CAD build for the part. Positions are in the model's coordinates, mm. A direction names the side the tool comes from. Round coordinates to 2 decimals unless told otherwise and drop trailing zeros. Loops run counter-clockwise (first coordinate to the right, second up) from the corner with the lowest first, then second, coordinate; pieces in that order, holes last.
```python
from build123d import *
from build123d.topology import SkipClean

# Parameters (mm, degrees)
BOSS_EXTRUDE1_DEPTH             = 10
BOSS_EXTRUDE2_DEPTH             = 1
BOSS_EXTRUDE3_DEPTH             = 7
CUT_EXTRUDE1_REACH              = 22.186
CUT_EXTRUDE2_REACH              = 22.166
BOSS_EXTRUDE4_REACH             = 24.566
BOSS_EXTRUDE4_END_RADIUS        = 3.5
SKETCH6_W                       = 5
SKETCH6_H                       = 3.45
SKETCH6_W_2                     = 3.2
SKETCH6_H_2                     = 1.65
BOSS_EXTRUDE4_DIRECTION_2_DEPTH = 19
CUT_EXTRUDE3_REACH              = 32.254
CUT_EXTRUDE4_REACH              = 32.254
CUT_EXTRUDE5_REACH              = 30.604


with BuildPart() as part:
    # Sketch1 → Boss-Extrude1 (new body)
    with BuildSketch(Plane(origin=(0, 0, 0), x_dir=(1, 0, 0), z_dir=(0, 1, 0))):
        with BuildLine():
            Line((-7.414489618, 1.20663528), (-4.430578599, 0.893013594))
            ThreePointArc((-4.430578599, 0.893013594), (-4.262003609, 0.936193276), (-4.162443929, 1.078916372))
            ThreePointArc((-4.162443929, 1.078916372), (-3.040559159, 3.040559159), (-1.078916372, 4.162443929))
            ThreePointArc((-1.078916372, 4.162443929), (-0.936193276, 4.262003609), (-0.893013594, 4.430578599))
            Line((-0.893013594, 4.430578599), (-1.20663528, 7.414489618))
            Line((-1.20663528, 7.414489618), (-0.361291669, 7.503338812))
            Line((-0.361291669, 7.503338812), (-0.047669983, 4.519427793))
            ThreePointArc((-0.047669983, 4.519427793), (0.02961483, 4.363514132), (0.189918705, 4.29580387))
            ThreePointArc((0.189918705, 4.29580387), (3.856330167, 1.902292734), (3.524282323, -2.463622152))
            Line((3.524282323, -2.463622152), (2.947715037, -1.887054865))
            ThreePointArc((2.947715037, -1.887054865), (-2.474873734, 2.474873734), (1.887054865, -2.947715037))
            Line((1.887054865, -2.947715037), (2.463622152, -3.524282323))
            ThreePointArc((2.463622152, -3.524282323), (-1.902292734, -3.856330167), (-4.29580387, -0.189918705))
            ThreePointArc((-4.29580387, -0.189918705), (-4.363514132, -0.02961483), (-4.519427793, 0.047669983))
            Line((-4.519427793, 0.047669983), (-7.503338812, 0.361291669))
            Line((-7.503338812, 0.361291669), (-7.414489618, 1.20663528))
        make_face()
    extrude(amount=-BOSS_EXTRUDE1_DEPTH)

    # Sketch2 → Boss-Extrude2 (add)
    with BuildSketch(Plane(origin=(0, -8.25, 0), x_dir=(-1, 0, 0), z_dir=(0, -1, 0))):
        with BuildLine():
            Line((-1.887054865, -2.947715037), (-1.15601211, -2.216672281))
            ThreePointArc((-1.15601211, -2.216672281), (1.767766953, 1.767766953), (-2.216672281, -1.15601211))
            Line((-2.216672281, -1.15601211), (-2.947715037, -1.887054865))
            ThreePointArc((-2.947715037, -1.887054865), (2.474873734, 2.474873734), (-1.887054865, -2.947715037))
        make_face()
    extrude(amount=BOSS_EXTRUDE2_DEPTH)

    # Sketch3 → Boss-Extrude3 (add)
    with SkipClean():  # the faces are left unmerged after this step: merging them gives an invalid solid
        with BuildSketch(Plane.XZ.offset(10)):
            with BuildLine():
                Line((-7.503338812, -0.361291669), (-3.499493713, 0.059529408))
                ThreePointArc((-3.499493713, 0.059529408), (-3.480826634, -0.365849621), (-3.41064452, -0.785814203))
                Line((-3.41064452, -0.785814203), (-7.414489618, -1.20663528))
                Line((-7.414489618, -1.20663528), (-7.503338812, -0.361291669))
            make_face()
            with BuildLine():
                Line((-1.20663528, -7.414489618), (-0.785814203, -3.41064452))
                ThreePointArc((-0.785814203, -3.41064452), (-0.365849621, -3.480826634), (0.059529408, -3.499493713))
                Line((0.059529408, -3.499493713), (-0.361291669, -7.503338812))
                Line((-0.361291669, -7.503338812), (-1.20663528, -7.414489618))
            make_face()
        extrude(amount=BOSS_EXTRUDE3_DEPTH)

    # Sketch4 → Cut-Extrude1 (cut, up to next)
    with BuildSketch(Plane(origin=(-0.044424597, 0, 0.422671806), x_dir=(0.9945218953682731, 0, 0.10452846326765693), z_dir=(-0.10452846326765693, 0, 0.9945218953682731)), mode=Mode.PRIVATE) as cut_extrude1_sk1:
        with BuildLine():
            Line((-4.499652764, 0), (-6.450238257, 0))
            ThreePointArc((-6.450238257, 0), (-7.174298022, -0.310262762), (-7.449060221, -1.048525086))
            Line((-7.449060221, -1.048525086), (-6.720325459, -16.048525086))
            ThreePointArc((-6.720325459, -16.048525086), (-6.411240733, -16.724059765), (-5.721503495, -17))
            Line((-5.721503495, -17), (-3.474100603, -17))
            Line((-3.474100603, -17), (-3.474100603, -18.237576525))
            Line((-3.474100603, -18.237576525), (-8.636241127, -18.237576525))
            Line((-8.636241127, -18.237576525), (-8.636241127, 0.642542217))
            Line((-8.636241127, 0.642542217), (-4.499652764, 0.642542217))
            Line((-4.499652764, 0.642542217), (-4.499652764, 0))
        make_face()
    cut_extrude1_tool1 = extrude(cut_extrude1_sk1.sketch, amount=-CUT_EXTRUDE1_REACH, mode=Mode.PRIVATE) & part.part
    add(cut_extrude1_tool1.solids().sort_by_distance((-7.422183, -10.016233, -0.352762))[0], mode=Mode.SUBTRACT)

    # Sketch5 → Cut-Extrude2 (cut, up to next)
    with BuildSketch(Plane(origin=(0.422671806, 0, -0.044424597), x_dir=(-0.10452846326764693, 0, -0.9945218953682741), z_dir=(0.9945218953682741, 0, -0.10452846326764693)), mode=Mode.PRIVATE) as cut_extrude2_sk1:
        with BuildLine():
            Line((4.499652764, 0), (6.39817036, 0))
            ThreePointArc((6.39817036, 0), (7.158143292, -0.325651711), (7.446533622, -1.100531645))
            Line((7.446533622, -1.100531645), (6.7226182, -16.001332189))
            ThreePointArc((6.7226182, -16.001332189), (6.398202955, -16.710373204), (5.674254938, -17))
            Line((5.674254938, -17), (3.474100603, -17))
            Line((3.474100603, -17), (3.474100603, -17.961134023))
            Line((3.474100603, -17.961134023), (9.689471059, -17.961134023))
            Line((9.689471059, -17.961134023), (9.520710585, 0.644708136))
            Line((9.520710585, 0.644708136), (4.499652764, 0.644708136))
            Line((4.499652764, 0.644708136), (4.499652764, 0))
        make_face()
    cut_extrude2_tool1 = extrude(cut_extrude2_sk1.sketch, amount=-CUT_EXTRUDE2_REACH, mode=Mode.PRIVATE) & part.part
    add(cut_extrude2_tool1.solids().sort_by_distance((-0.417746, -9.418745, -8.040463))[0], mode=Mode.SUBTRACT)

    # Boss-Extrude4: up to this cylinder (the profile starts outside it)
    with SkipClean():  # the faces are left unmerged after this step: merging them gives an invalid solid
        boss_extrude4_end = Plane(origin=(0, -1.260747, 0), z_dir=(0, 1, 0)) * Cylinder(BOSS_EXTRUDE4_END_RADIUS, 57.132, mode=Mode.PRIVATE)
        # Sketch6 → Boss-Extrude4 (add, up to the surface)
        with BuildSketch(Plane(origin=(3.040559159, 0, 3.040559159), x_dir=(0.7071067811865511, 0, -0.707106781186544), z_dir=(0.707106781186544, 0, 0.7071067811865511)), mode=Mode.PRIVATE) as boss_extrude4_sk1:
            with Locations((0, -2.925)):
                Rectangle(SKETCH6_W, SKETCH6_H)
            with Locations((0, -2.925)):
                Rectangle(SKETCH6_W_2, SKETCH6_H_2, mode=Mode.SUBTRACT)
        boss_extrude4_tool1 = extrude(boss_extrude4_sk1.sketch, amount=-BOSS_EXTRUDE4_REACH, mode=Mode.PRIVATE) - boss_extrude4_end
        add(boss_extrude4_tool1.solids().sort_by_distance((3.040559, -1.260747, 3.040559))[0])

    # Sketch6 → Boss-Extrude4 direction 2 (add)
    with SkipClean():  # the faces are left unmerged after this step: merging them gives an invalid solid
        with BuildSketch(Plane(origin=(3.040559159, 0, 3.040559159), x_dir=(0.7071067811865511, 0, -0.707106781186544), z_dir=(0.707106781186544, 0, 0.7071067811865511))):
            with Locations((0, -2.925)):
                Rectangle(SKETCH6_W, SKETCH6_H)
            with Locations((0, -2.925)):
                Rectangle(SKETCH6_W_2, SKETCH6_H_2, mode=Mode.SUBTRACT)
        extrude(amount=BOSS_EXTRUDE4_DIRECTION_2_DEPTH)

    # Sketch7 → Cut-Extrude3 (cut, up to next)
    with BuildSketch(Plane(origin=(0, -1.2, 0), x_dir=(1, 0, 0), z_dir=(0, 1, 0)), mode=Mode.PRIVATE) as cut_extrude3_sk1:
        with BuildLine():
            Line((15.344217152, -17.606958852), (13.965358928, -16.228100628))
            ThreePointArc((13.965358928, -16.228100628), (13.511374439, -15.132085117), (13.965358928, -14.036069607))
            Line((13.965358928, -14.036069607), (14.036069607, -13.965358928))
            ThreePointArc((14.036069607, -13.965358928), (15.132085117, -13.511374439), (16.228100628, -13.965358928))
            Line((16.228100628, -13.965358928), (17.606958852, -15.344217152))
            Line((17.606958852, -15.344217152), (15.344217152, -17.606958852))
        make_face()
    cut_extrude3_tool1 = extrude(cut_extrude3_sk1.sketch, amount=-CUT_EXTRUDE3_REACH, mode=Mode.PRIVATE) & part.part
    # Sketch7 → Cut-Extrude3 (cut, up to next)
    with BuildSketch(Plane(origin=(0, -1.2, 0), x_dir=(1, 0, 0), z_dir=(0, 1, 0)), mode=Mode.PRIVATE) as cut_extrude3_sk2:
        Polygon((8.379215357, -10.641957057), (10.641957057, -8.379215357), (13.116830791, -10.854089091), (10.854089091, -13.116830791), align=None)
    cut_extrude3_tool2 = extrude(cut_extrude3_sk2.sketch, amount=-CUT_EXTRUDE3_REACH, mode=Mode.PRIVATE) & part.part
    # Sketch7 → Cut-Extrude3 (cut, up to next)
    with BuildSketch(Plane(origin=(0, -1.2, 0), x_dir=(1, 0, 0), z_dir=(0, 1, 0)), mode=Mode.PRIVATE) as cut_extrude3_sk3:
        Polygon((3.924442636, -6.187184335), (6.187184335, -3.924442636), (8.591347391, -6.328605692), (6.328605692, -8.591347391), align=None)
    cut_extrude3_tool3 = extrude(cut_extrude3_sk3.sketch, amount=-CUT_EXTRUDE3_REACH, mode=Mode.PRIVATE) & part.part
    add(cut_extrude3_tool1.solids().sort_by_distance((15.338807, -1.2, 15.338807))[0], mode=Mode.SUBTRACT)
    add(cut_extrude3_tool2.solids().sort_by_distance((10.748023, -1.2, 10.748023))[0], mode=Mode.SUBTRACT)
    add(cut_extrude3_tool3.solids().sort_by_distance((6.257895, -1.2, 6.257895))[0], mode=Mode.SUBTRACT)

    # Cut-Extrude4: up to this face of the body (flat: up to its plane)
    cut_extrude4_end = Plane(part.part.faces().sort_by_distance((9.75807358, -4.65, 9.75807358))[0])
    # Sketch8 → Cut-Extrude4 (cut, up to the picked face)
    with BuildSketch(Plane(origin=(0, -1.2, 0), x_dir=(1, 0, 0), z_dir=(0, 1, 0)), mode=Mode.PRIVATE) as cut_extrude4_sk1:
        with BuildLine():
            Line((1.887054865, -2.947715037), (2.463622152, -3.524282323))
            ThreePointArc((2.463622152, -3.524282323), (2.122539393, -3.739629196), (1.762778319, -3.922067388))
            Line((1.762778319, -3.922067388), (1.894971957, -4.082617205))
            ThreePointArc((1.894971957, -4.082617205), (2.256834016, -4.264215104), (2.634518611, -4.118351149))
            Line((2.634518611, -4.118351149), (4.118351149, -2.634518611))
            ThreePointArc((4.118351149, -2.634518611), (4.264215104, -2.256834016), (4.082617205, -1.894971957))
            Line((4.082617205, -1.894971957), (3.922067388, -1.762778319))
            ThreePointArc((3.922067388, -1.762778319), (3.739629196, -2.122539393), (3.524282323, -2.463622152))
            Line((3.524282323, -2.463622152), (2.947715037, -1.887054865))
            ThreePointArc((2.947715037, -1.887054865), (2.474873734, -2.474873734), (1.887054865, -2.947715037))
        make_face()
    cut_extrude4_tool1 = split(extrude(cut_extrude4_sk1.sketch, amount=-CUT_EXTRUDE4_REACH, mode=Mode.PRIVATE), bisect_by=cut_extrude4_end, keep=Keep.BOTH, mode=Mode.PRIVATE)
    add(cut_extrude4_tool1.solids().sort_by(Axis((2.984609, -1.2, 2.984609), (0, -1, 0)))[0], mode=Mode.SUBTRACT)

    # Sketch9 → Cut-Extrude5 (cut, up to next)
    with BuildSketch(Plane.XZ.offset(4.65), mode=Mode.PRIVATE) as cut_extrude5_sk1:
        Polygon((9.75807358, 12.02081528), (12.02081528, 9.75807358), (17.606958852, 15.344217152), (15.344217152, 17.606958852), align=None)
    cut_extrude5_tool1 = extrude(cut_extrude5_sk1.sketch, amount=-CUT_EXTRUDE5_REACH, mode=Mode.PRIVATE) & part.part
    # Sketch9 → Cut-Extrude5 (cut, up to next)
    with BuildSketch(Plane.XZ.offset(4.65), mode=Mode.PRIVATE) as cut_extrude5_sk2:
        Polygon((8.485281374, 10.748023074), (10.748023074, 8.485281374), (8.27314934, 6.01040764), (6.01040764, 8.27314934), align=None)
    cut_extrude5_tool2 = extrude(cut_extrude5_sk2.sketch, amount=-CUT_EXTRUDE5_REACH, mode=Mode.PRIVATE) & part.part
    # Sketch9 → Cut-Extrude5 (cut, up to next)
    with BuildSketch(Plane.XZ.offset(4.65), mode=Mode.PRIVATE) as cut_extrude5_sk3:
        Polygon((2.952170811, 5.214912511), (5.214912511, 2.952170811), (7.000357134, 4.737615434), (4.737615434, 7.000357134), align=None)
    cut_extrude5_tool3 = extrude(cut_extrude5_sk3.sketch, amount=-CUT_EXTRUDE5_REACH, mode=Mode.PRIVATE) & part.part
    add(cut_extrude5_tool1.solids().sort_by_distance((13.682516, -4.65, 13.682516))[0], mode=Mode.SUBTRACT)
    add(cut_extrude5_tool2.solids().sort_by_distance((8.379215, -4.65, 8.379215))[0], mode=Mode.SUBTRACT)
    add(cut_extrude5_tool3.solids().sort_by_distance((4.976264, -4.65, 4.976264))[0], mode=Mode.SUBTRACT)


solid = part.part
```
Item 1: Cut at D-D, the plane y = -7.25. Give the cut face in (x, z).
Answers follow:
outline: (-7.15, -0.32) - (-7.06, -1.17) - (-4.43, -0.89) arc R0.25 cw to (-4.16, -1.08) arc R4.3 ccw to (-1.08, -4.16) arc R0.25 cw to (-0.89, -4.43) - (-1.17, -7.06) - (-0.32, -7.15) - (-0.05, -4.52) arc R0.25 cw to (0.19, -4.3) arc R4.3 ccw to (3.52, 2.46) - (2.95, 1.89) arc R3.5 cw (long way) to (1.89, 2.95) - (2.46, 3.52) arc R4.3 ccw to (-4.3, 0.19) arc R0.25 cw to (-4.52, -0.05) - close
Item 2: Probe line 1 (Y direction, x = 10.75, z = 13.25); line 2 (Z direction, x = 0, y = -9); line 3 (Y direction, x = 5.5, z = 7.25). List the from-to ranges inside material, lowest first.
Answers follow:
line 1: y = -4.65 to -1.2
line 2: z = -4.4 to -2.5, 2.5 to 4.3
line 3: y = -4.65 to -3.75
Item 3: 3-axis set-ups, long thin cutter, end or side, ignore diameter. For faces 1 (the flat face through (10.68, -2.9, 8.42)), 2 (the flat face through (-3, -8.25, 0)), 3 (the flat face through (5.885, -4.206, 5.853)): which of +Z, -Z, +X, -X, +Y, -Y reach the whole face in a straight line?
Answers follow:
face 1: none
face 2: +Y
face 3: +Y, -Y
Item 4: Cut at C-C, the plane y = -5. Give the cut face in (x, z).
Answers follow:
outline: (-7.26, -0.34) - (-7.17, -1.18) - (-4.43, -0.89) arc R0.25 cw to (-4.16, -1.08) arc R4.3 ccw to (-1.08, -4.16) arc R0.25 cw to (-0.89, -4.43) - (-1.18, -7.17) - (-0.34, -7.26) - (-0.05, -4.52) arc R0.25 cw to (0.19, -4.3) arc R4.3 ccw to (3.52, 2.46) - (2.95, 1.89) arc R3.5 cw (long way) to (1.89, 2.95) - (2.46, 3.52) arc R4.3 ccw to (-4.3, 0.19) arc R0.25 cw to (-4.52, -0.05) - close
Item 5: Cut at B-B, the plane y = -15. Give the cut face in (x, z).
Answers follow:
outline: (-6.78, -0.29) - (-6.69, -1.13) - (-3.41, -0.79) arc R3.5 cw to (-3.5, 0.06) - close; (-1.13, -6.69) - (-0.29, -6.78) - (0.06, -3.5) arc R3.5 cw to (-0.79, -3.41) - close
Item 6: Two-plate mould, pull along Z, no slides. Class faces 4 (the flat face through (-0.5, -17, -4.5)), 5 (the cylindrical face through (13.51, -1.64, 15.15)), 6 (the flat face through (-0.74, -8.45, -7.05)): released by +Z, released by -Z, zero draft, split by the parting line, or undercut.
Answers follow:
face 4: zero draft
face 5: undercut
face 6: released by -Z
Item 7: Cut at A-A, the plane y = -10.75. Give the cut face in (x, z), plus the area to 3 significant figures.
Answers follow:
outline: (-6.98, -0.31) - (-6.9, -1.15) - (-3.41, -0.79) arc R3.5 cw to (-3.5, 0.06) - close; (-1.15, -6.9) - (-0.31, -6.98) - (0.06, -3.5) arc R3.5 cw to (-0.79, -3.41) - close
area: 5.93 mm2
Item 8: Flat gauge pins, fed straight in: P1, Ø4, axis at x = 0.5, y = -3, coming from the -Z side; P2, Ø4, axis at x = 10.5, z = 10.5, coming from the +Y side; P3, Ø12, axis at x = 12.5, z = 1, coming from the -Y side. Where does each tip first touch, or does it go through?
Answers follow:
P1: stops at z = -7.45
P2: stops at y = -1.2
P3: stops at y = -4.65
